Source: three-view drawing plus pictorial views. Frame: mm from the lowest corner of the part. A direction names the side the tool comes from. Give positions to 0.01 mm unless a question says otherwise; leave off trailing zeros. Loops run counter-clockwise (first coordinate to the right, second up) from the corner with the lowest first, then second, coordinate; pieces in that order, holes last. Notation, with made-up numbers: (81.5, 80.25) -> (131.5, 80.25) arc R17 ccw to (131.5, 91.25) -> close; hole circle Ø9 at (-30, 8.25). An arc over 180 degrees is marked (long way). Put each result on its own line as item: value.
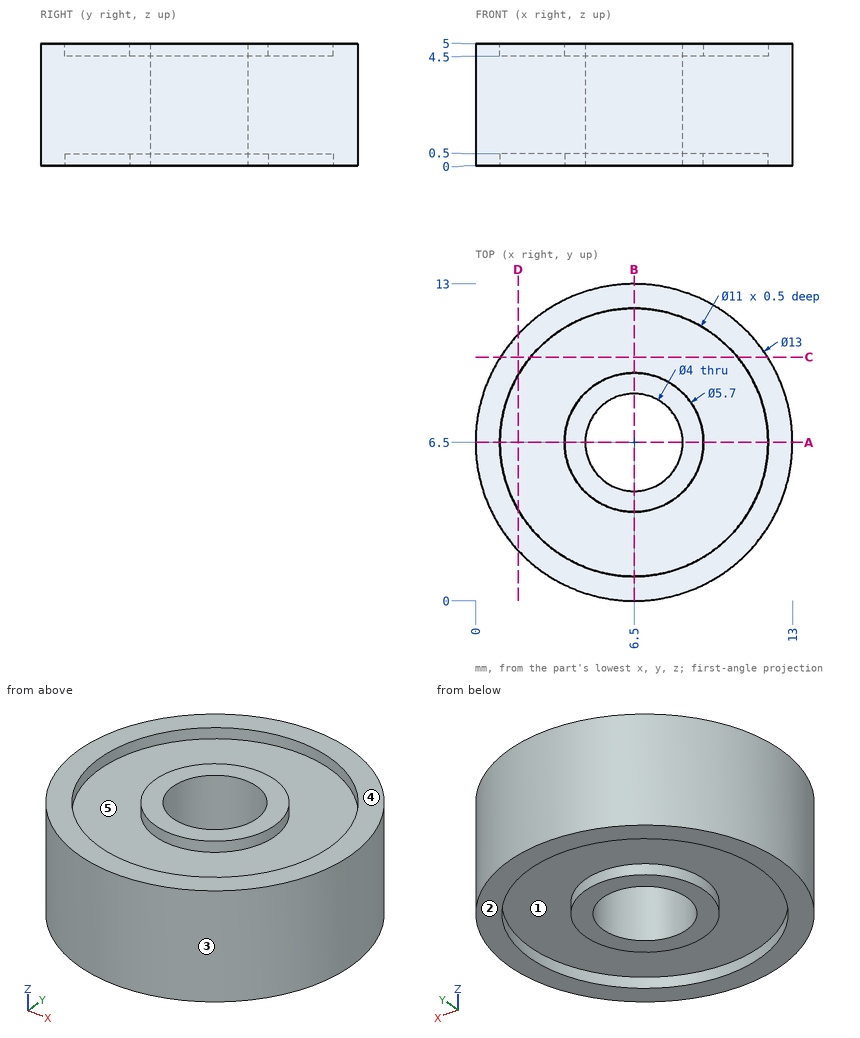
(1) Line query: probe 1 along Y at (x, z) = (6.5, 0.1); probe 2 along X at (y, z) = (9, 4.55); probe 3 along Y at (x, z) = (6.5, 3.2). Output: solid intervals per line, ascending. Write a range as from..to.
Calculated:
probe 1: y = 0..1, 3.65..4.5, 8.5..9.35, 12..13
probe 2: x = 0.5..1.6, 5.13..7.87, 11.4..12.5
probe 3: y = 0..4.5, 8.5..13
(2) Reachability of the marked faces 4 and 5 from +Z, -Z, +X, -X, +Y, -Y: full face, straight path, thin tool, end or side. Return the list, or none.
Calculated:
face 4: +Z, +X, -X, +Y, -Y
face 5: +Z
(3) Section D-D on x = 1.75. Return loops of the section in (y, z).
Calculated:
outline: (2.06, 0) -> (3.73, 0) -> (3.73, 0.5) -> (9.27, 0.5) -> (9.27, 0) -> (10.94, 0) -> (10.94, 5) -> (9.27, 5) -> (9.27, 4.5) -> (3.73, 4.5) -> (3.73, 5) -> (2.06, 5) -> close
(4) Section C-C on y = 10. Return loops of the section in (x, z).
Calculated:
outline: (1.02, 0) -> (2.26, 0) -> (2.26, 0.5) -> (10.74, 0.5) -> (10.74, 0) -> (11.98, 0) -> (11.98, 5) -> (10.74, 5) -> (10.74, 4.5) -> (2.26, 4.5) -> (2.26, 5) -> (1.02, 5) -> close
(5) Section A-A on y = 6.5. Return loops of the section in (x, z), then the cut area to 3 significant figures.
Calculated:
outline: (0, 0) -> (1, 0) -> (1, 0.5) -> (3.65, 0.5) -> (3.65, 0) -> (4.5, 0) -> (4.5, 5) -> (3.65, 5) -> (3.65, 4.5) -> (1, 4.5) -> (1, 5) -> (0, 5) -> close; (8.5, 0) -> (9.35, 0) -> (9.35, 0.5) -> (12, 0.5) -> (12, 0) -> (13, 0) -> (13, 5) -> (12, 5) -> (12, 4.5) -> (9.35, 4.5) -> (9.35, 5) -> (8.5, 5) -> close
area: 39.7 mm²
(6) First-contact query: P1, Ø1, axis at x = 5, y = 7.5, coming from the +Z side; P2, Ø3, axis at x = 10.5, z = 3, coming from the -Y side. Flat tips, straight axial feed; report the tip coordinate or a pass-through.
Calculated:
P1: stops at z = 5
P2: stops at y = 0.5
(7) Draft query along Y for the marked faces 1, 2 and 3. Return one class per face: released by +Y, released by -Y, zero draft, split by the parting line, or undercut.
Calculated:
face 1: undercut
face 2: zero draft
face 3: split by the parting line
